Could you check a few things on this model? Use its own coordinates, in mm. A direction names the side the tool comes from. Round coordinates to 2 decimals unless told otherwise and drop trailing zeros. Write each loop counter-clockwise with the first axis right and the second up, starting at its lowest first coordinate (ties: lowest second). Pieces come first, ordered by that corner, then holes. Notation, with made-up numbers: (-39, 83) -> (-21, 83) arc R8 ccw to (-21, 93) -> close; hole circle Ø10 at (65.25, 70). An arc over 180 degrees is marked (long way). Answer in a Markdown table with one row per item.
from build123d import *

# Parameters (mm, degrees)
SKETCH2_R           = 2.3
BOSS_EXTRUDE1_DEPTH = 4


with BuildPart() as part:
    # Sketch2 → Boss-Extrude1 (new body)
    with BuildSketch(Plane(origin=(0, 0, 0), x_dir=(1, 0, 0), z_dir=(0, 1, 0))):
        with BuildLine():
            Line((-2.784735434, -5.571506186), (-2.425826245, -7.32540615))
            ThreePointArc((-2.425826245, -7.32540615), (-2.065386908, -7.708128878), (-1.561875921, -7.556900941))
            Line((-1.561875921, -7.556900941), (-0.374101464, -6.217433611))
            ThreePointArc((-0.374101464, -6.217433611), (0, -6.049168588), (0.374101464, -6.217433611))
            Line((0.374101464, -6.217433611), (1.561875921, -7.556900941))
            ThreePointArc((1.561875921, -7.556900941), (2.065386908, -7.708128878), (2.425826245, -7.32540615))
            Line((2.425826245, -7.32540615), (2.784735434, -5.571506186))
            ThreePointArc((2.784735434, -5.571506186), (3.024584294, -5.238733669), (3.432698177, -5.197404722))
            Line((3.432698177, -5.197404722), (5.131074696, -5.763530228))
            ThreePointArc((5.131074696, -5.763530228), (5.64274197, -5.64274197), (5.763530228, -5.131074696))
            Line((5.763530228, -5.131074696), (5.197404722, -3.432698177))
            ThreePointArc((5.197404722, -3.432698177), (5.238733669, -3.024584294), (5.571506186, -2.784735434))
            Line((5.571506186, -2.784735434), (7.32540615, -2.425826245))
            ThreePointArc((7.32540615, -2.425826245), (7.708128878, -2.065386908), (7.556900941, -1.561875921))
            Line((7.556900941, -1.561875921), (6.217433611, -0.374101464))
            ThreePointArc((6.217433611, -0.374101464), (6.049168588, 0), (6.217433611, 0.374101464))
            Line((6.217433611, 0.374101464), (7.556900941, 1.561875921))
            ThreePointArc((7.556900941, 1.561875921), (7.708128878, 2.065386908), (7.32540615, 2.425826245))
            Line((7.32540615, 2.425826245), (5.571506186, 2.784735434))
            ThreePointArc((5.571506186, 2.784735434), (5.238733669, 3.024584294), (5.197404722, 3.432698177))
            Line((5.197404722, 3.432698177), (5.763530228, 5.131074696))
            ThreePointArc((5.763530228, 5.131074696), (5.64274197, 5.64274197), (5.131074696, 5.763530228))
            Line((5.131074696, 5.763530228), (3.432698177, 5.197404722))
            ThreePointArc((3.432698177, 5.197404722), (3.024584294, 5.238733669), (2.784735434, 5.571506186))
            Line((2.784735434, 5.571506186), (2.425826245, 7.32540615))
            ThreePointArc((2.425826245, 7.32540615), (2.065386908, 7.708128878), (1.561875921, 7.556900941))
            Line((1.561875921, 7.556900941), (0.374101464, 6.217433611))
            ThreePointArc((0.374101464, 6.217433611), (0, 6.049168588), (-0.374101464, 6.217433611))
            Line((-0.374101464, 6.217433611), (-1.561875921, 7.556900941))
            ThreePointArc((-1.561875921, 7.556900941), (-2.065386908, 7.708128878), (-2.425826245, 7.32540615))
            Line((-2.425826245, 7.32540615), (-2.784735434, 5.571506186))
            ThreePointArc((-2.784735434, 5.571506186), (-3.024584294, 5.238733669), (-3.432698177, 5.197404722))
            Line((-3.432698177, 5.197404722), (-5.131074696, 5.763530228))
            ThreePointArc((-5.131074696, 5.763530228), (-5.64274197, 5.64274197), (-5.763530228, 5.131074696))
            Line((-5.763530228, 5.131074696), (-5.197404722, 3.432698177))
            ThreePointArc((-5.197404722, 3.432698177), (-5.238733669, 3.024584294), (-5.571506186, 2.784735434))
            Line((-5.571506186, 2.784735434), (-7.32540615, 2.425826245))
            ThreePointArc((-7.32540615, 2.425826245), (-7.708128878, 2.065386908), (-7.556900941, 1.561875921))
            Line((-7.556900941, 1.561875921), (-6.217433611, 0.374101464))
            ThreePointArc((-6.217433611, 0.374101464), (-6.049168588, 0), (-6.217433611, -0.374101464))
            Line((-6.217433611, -0.374101464), (-7.556900941, -1.561875921))
            ThreePointArc((-7.556900941, -1.561875921), (-7.708128878, -2.065386908), (-7.32540615, -2.425826245))
            Line((-7.32540615, -2.425826245), (-5.571506186, -2.784735434))
            ThreePointArc((-5.571506186, -2.784735434), (-5.238733669, -3.024584294), (-5.197404722, -3.432698177))
            Line((-5.197404722, -3.432698177), (-5.763530228, -5.131074696))
            ThreePointArc((-5.763530228, -5.131074696), (-5.64274197, -5.64274197), (-5.131074696, -5.763530228))
            Line((-5.131074696, -5.763530228), (-3.432698177, -5.197404722))
            ThreePointArc((-3.432698177, -5.197404722), (-3.024584294, -5.238733669), (-2.784735434, -5.571506186))
        make_face()
        with Locations(Location((0, 0, 0), (0, 0, 270))):
            Circle(SKETCH2_R, mode=Mode.SUBTRACT)
    extrude(amount=-BOSS_EXTRUDE1_DEPTH)


solid = part.part
1) For pin 1 (1 mm diameter, centred on x = 6, y = -2, fed in from +Z); pin 2 (2 mm diameter, centred on x = 5, y = -2.5, fed in from -Z), each with a flat end and sliding along its axis, tell me the tip position at first contact or that it passes through.
Findings:
| item | result |
|---|---|
| pin 1 | stops at z = 5.74 |
| pin 2 | stops at z = -5.79 |
2) Thinking about a two-plate mould opening in X: for faces 1 (the face through (-2.073, -1.972, 7.706)), 2 (the face through (6.436, -1.972, 2.608)), 3 (the face through (2, 0, -2)), which applies, +X half, -X half, draft (parallel to the pull), parting line (faces both ways), or undercut?
Findings:
| item | result |
|---|---|
| face 1 | undercut |
| face 2 | +X half |
| face 3 | draft |
3) Imagine slicing it at B-B, the plane z = 0. Please give me the cut outline in (x, y), plus the area to 3 significant figures.
Findings:
| item | result |
|---|---|
| outline | (-6.05, -4) -> (-2.3, -4) -> (-2.3, 0) -> (-6.05, 0) -> close; (2.3, -4) -> (6.05, -4) -> (6.05, 0) -> (2.3, 0) -> close |
| area | 30.0 mm^2 |
4) Please list where these lines run through material, in increasing order: line 1 (X direction, y = -1.45, z = 0); line 2 (X direction, y = -3.3, z = -2); line 3 (Z direction, x = -6.25, y = -1.5).
Findings:
| item | result |
|---|---|
| line 1 | x = -6.05 to -2.3, 2.3 to 6.05 |
| line 2 | x = -7.72 to -1.14, 1.14 to 7.72 |
| line 3 | z = -2.65 to -0.4, 0.4 to 2.65 |
5) Imagine slicing it at D-D, the plane x = -3.25. Please give me the cut outline in (y, z).
Findings:
| item | result |
|---|---|
| outline | (-4, -5.17) -> (0, -5.17) -> (0, 5.17) -> (-4, 5.17) -> close |
6) Imagine slicing it at C-C, the plane x = 3. Please give me the cut outline in (y, z), plus the area to 3 significant figures.
Findings:
| item | result |
|---|---|
| outline | (-4, -5.25) -> (0, -5.25) -> (0, 5.25) -> (-4, 5.25) -> close |
| area | 42.0 mm^2 |
7) For faces 4 (the face through (-6.9, -1.97, -0.98)), 5 (the face through (4.27, -1.972, 5.477)), 6 (the face through (5.484, -1.972, 4.294)), 7 (the face through (-4.27, -1.972, -5.477)), which set-ups out of +Z, -Z, +X, -X, +Y, -Y let a thin tool reach every point of the face, with its end or its side?
Findings:
| item | result |
|---|---|
| face 4 | -X, +Y, -Y |
| face 5 | +Z, +Y, -Y |
| face 6 | +X, +Y, -Y |
| face 7 | -Z, +Y, -Y |
8) Imagine slicing it at A-A, the plane x = 0. Please give me the cut outline in (y, z).
Findings:
| item | result |
|---|---|
| outline | (-4, -6.05) -> (0, -6.05) -> (0, -2.3) -> (-4, -2.3) -> close; (-4, 2.3) -> (0, 2.3) -> (0, 6.05) -> (-4, 6.05) -> close |
